Geometry: see drawing. Coordinates: mm, zero at the bounding-box minimum. A direction names the side the tool comes from. Round coordinates to 2 decimals unless told otherwise and drop trailing zeros. Order: outer loops, then holes, each group sorted by start corner. A loop starts at its lowest first (then second) coordinate and runs counter-clockwise, first axis right, second up. Notation, with made-up numbers: (-15.75, -17) -> (-5.75, -17) arc R19 ccw to (-5.75, 11) -> close; hole circle Ø11 at (-27.75, 64). An arc over 180 degrees is marked (long way). One line per item, written item: value. Start each with the question number.
1) Section D-D (y = 4.5). Return the cut outline in (x, z).
2) Reachability of the marked faces 1 and 2 from +Z, -Z, +X, -X, +Y, -Y: full face, straight path, thin tool, end or side. Return the list, or none.
3) Section B-B (y = 14). Return the cut outline in (x, z), and give its area (3 significant figures).
4) Ray query, L1, parallel to Y at x = 17.5, z = 25.5; L2, parallel to Z at x = 11, y = 12; L3, parallel to X at y = 14, z = 18. Return the intervals inside material, ascending.
5) Pin query (flat end, axial travel): P1, Ø11, axis at x = 10, z = 29, coming from the -Y side; P2, Ø14, axis at x = 19.5, y = 9, coming from the +Z side; P3, Ø2, axis at y = 19.5, z = 27, coming from the +X side; P4, Ø12, axis at x = 33, z = 8, coming from the -Y side. Return the tip coordinate at first contact, or that it passes through.
6) Section A-A (x = 10). Return the cut outline in (y, z).
7) Section C-C (z = 20). Return the cut outline in (x, y).
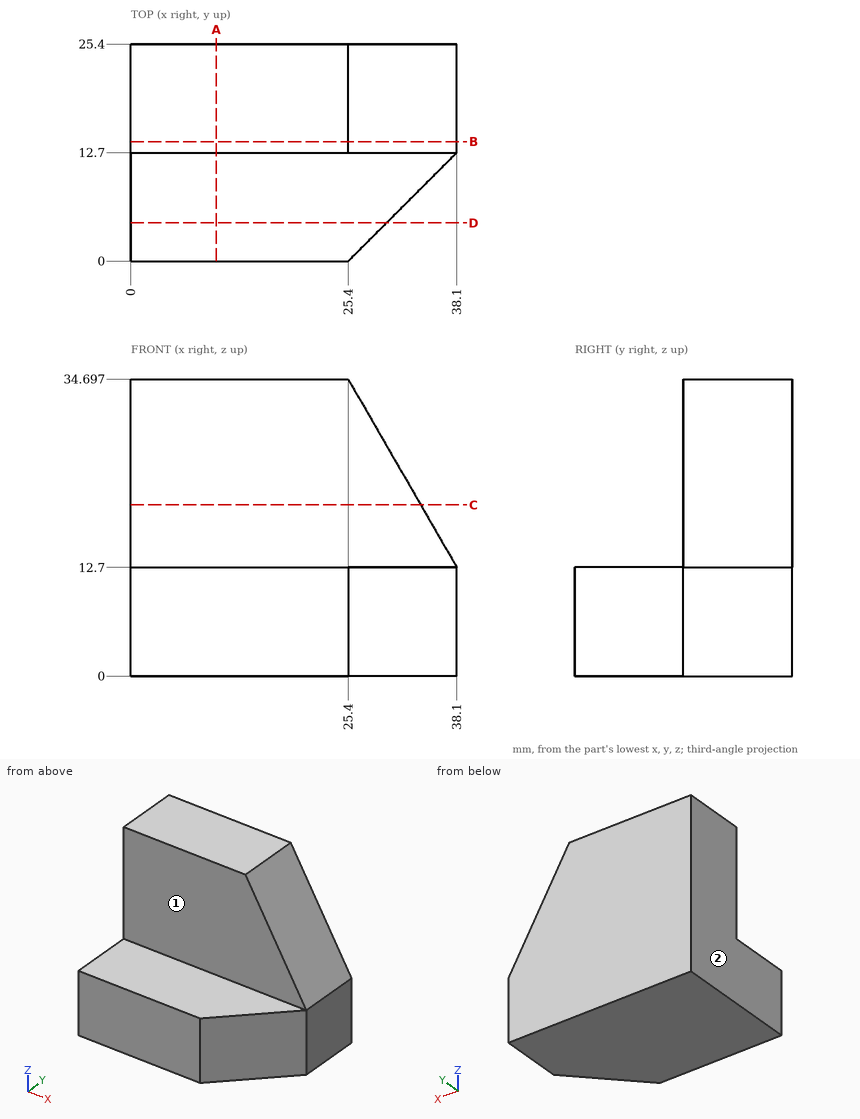
Findings:
1. outline: (0, 0) -> (29.9, 0) -> (29.9, 12.7) -> (0, 12.7) -> close
2. face 1: +Z, +X, -X, -Y
2. face 2: +Z, -Z, -X, +Y, -Y
3. outline: (0, 0) -> (38.1, 0) -> (38.1, 12.7) -> (25.4, 34.7) -> (0, 34.7) -> close
3. area: 1,180 mm2
4. L1: 12.7 to 25.4
4. L2: 0 to 12.7
4. L3: 0 to 35.04
5. P1: y = 12.7
5. P2: z = 34.7
5. P3: x = 30.42
5. P4: y = 1.6
6. outline: (0, 0) -> (25.4, 0) -> (25.4, 34.7) -> (12.7, 34.7) -> (12.7, 12.7) -> (0, 12.7) -> close
7. outline: (0, 12.7) -> (33.89, 12.7) -> (33.89, 25.4) -> (0, 25.4) -> close
